Model file for the job. Use its own axes, mm. Face numbers are marked on the shaded views. A direction names the side the tool comes from. Give positions to 0.01 mm unless a question says otherwise; leave off trailing zeros. Loops run counter-clockwise (first coordinate to the right, second up) from the corner with the lowest first, then second, coordinate; pieces in that order, holes last. Notation, with made-up numbers: (28, 73) - (82, 73) arc R20 cw to (82, 92) - close; hole circle Ø8 at (37.5, -25.75). An arc over 180 degrees is marked (long way). Answer as CSV lines item,"result". Start each with the question number.
Item 1: Saw through at B-B on x = -39. Give the cut face in (y, z).
Item 2: Pin check, flat tips, straight feed: pin 1 (8 mm diameter, centred on x = -13, z = -10.5, fed in from -Y); pin 2 (4 mm diameter, centred on x = -20.5, y = 15, fed in from +Z); pin 3 (4 mm diameter, centred on x = -27, z = 18.5, fed in from -Y); pin 4 (1.5 mm diameter, centred on y = 22.5, z = -10, fed in from -X). Stop position of each tip, or through.
Item 3: Saw through at C-C on z = 0. Give the cut face in (x, y).
Item 4: Tool access for the marked faces 4, 5 and 6: list every direction of +Z, -Z, +X, -X, +Y, -Y with a clear straight run to the whole face (end or side of a thin tool).
Item 5: Saw through at A-A on z = 11. Give the cut face in (x, y).
Item 6: Drill centre lines: L1, parallel to Z at x = -61, y = 6.25; L2, parallel to Y at x = -70, z = 10; L3, parallel to X at y = 9.75, z = 12.35. Where is each one in solid material? Low to high. Write a range as from..to.
Item 7: Saw through at D-D on y = 21. Give the cut face in (x, z), plus the area to 3 significant figures.
Item 8: Pull direction X, two halves, no side cores. Call the marked faces 1, 2 and 3: pulls with the +X half, pulls with the -X half, needs draft (parallel to the pull), parting line crosses it, or undercut.
from build123d import *

# Parameters (mm, degrees)
SKETCH1_W           = 30
SKETCH1_H           = 19.5
BOSS_EXTRUDE1_DEPTH = 70
BOSS_EXTRUDE2_DEPTH = 30
SKETCH7_W           = 48
SKETCH7_H           = 45
BOSS_EXTRUDE3_DEPTH = 5
CUT_EXTRUDE2_START  = -6
SKETCH8_R           = 9.75
CUT_EXTRUDE2_DEPTH  = 18
SKETCH9_R           = 4
CUT_EXTRUDE3_DEPTH  = 92.468915485
SKETCH10_R          = 9
CUT_EXTRUDE4_DEPTH  = 10
CUT_EXTRUDE6_START  = -6
CUT_EXTRUDE6_DEPTH  = 18
FILLET1_R           = 10


with BuildPart() as part:
    # Sketch1 → Boss-Extrude1 (new body)
    with BuildSketch(Plane(origin=(0, 0, 0), x_dir=(0, 0, -1), z_dir=(1, 0, 0))):
        with Locations((0, 9.75)):
            Rectangle(SKETCH1_W, SKETCH1_H)
    extrude(amount=-BOSS_EXTRUDE1_DEPTH)

    # Sketch6 → Boss-Extrude2 (add)
    with BuildSketch(Plane.XY.offset(15)):
        with BuildLine():
            Line((-70, 19.5), (-70, 0))
            ThreePointArc((-70, 0), (-79.75, 9.75), (-70, 19.5))
        make_face()
    extrude(amount=-BOSS_EXTRUDE2_DEPTH)

    # Sketch7 → Boss-Extrude3 (add)
    with BuildSketch(Plane(origin=(0, 19.5, 0), x_dir=(1, 0, 0), z_dir=(0, 1, 0))):
        with Locations((-24, 0)):
            Rectangle(SKETCH7_W, SKETCH7_H)
    extrude(amount=BOSS_EXTRUDE3_DEPTH)

    # Sketch8 → Cut-Extrude2 (cut)
    with BuildSketch(Plane.XY.offset(15).offset(CUT_EXTRUDE2_START)):
        with Locations((-70, 9.75)):
            Circle(SKETCH8_R)
    extrude(amount=-CUT_EXTRUDE2_DEPTH, mode=Mode.SUBTRACT)

    # Sketch9 → Cut-Extrude3 (cut, through all)
    with BuildSketch(Plane.XY.offset(15)):
        with Locations((-70, 9.75)):
            Circle(SKETCH9_R)
    extrude(amount=-CUT_EXTRUDE3_DEPTH, mode=Mode.SUBTRACT)

    # Sketch10 → Cut-Extrude4 (cut)
    with BuildSketch(Plane.XZ):
        with Locations(Location((-24, 0, 0), (0, 0, 270))):
            Circle(SKETCH10_R)
    extrude(amount=-CUT_EXTRUDE4_DEPTH, mode=Mode.SUBTRACT)

    # Sketch11 → Cut-Extrude6 (cut)
    with BuildSketch(Plane(origin=(0, 0, -15), x_dir=(-1, 0, 0), z_dir=(0, 0, -1)).offset(CUT_EXTRUDE6_START)):
        Polygon((66.561504355, 11.793709299), (45, 0), (70, 0), align=None)
    extrude(amount=-CUT_EXTRUDE6_DEPTH, mode=Mode.SUBTRACT)

    # Fillet1
    fillet1_edges = [part.edges().sort_by_distance(p)[0] for p in [
        (-60.344849532, 8.393324122, 0),
    ]]
    fillet(fillet1_edges, radius=FILLET1_R)


solid = part.part
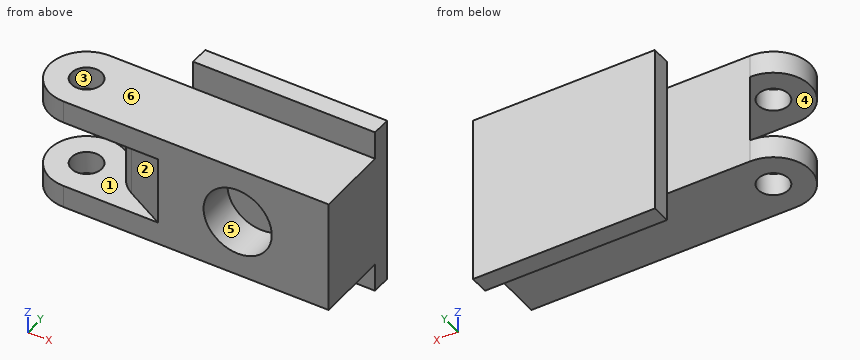
Responses:
1,outline,"(0, -15) - (19.5, -15) - (19.5, -22.5) - (24.5, -22.5) - (24.5, 22.5) - (19.5, 22.5) - (19.5, 15) - (0, 15) - close"
2,pin 1,"y = 0"
2,pin 2,"z = 15"
2,pin 3,"y = 19.5"
2,pin 4,"x = -48"
3,outline,"(-70, 19.5) arc R9.75 cw to (-60.55, 12.14) arc R10 ccw to (-55.65, 5.83) - (-45, 0) - (-33, 0) - (-33, 10) - (-15, 10) - (-15, 0) - (0, 0) - (0, 24.5) - (-48, 24.5) - (-48, 19.5) - close"
4,face 4,"-X, -Y"
4,face 5,"-Y"
4,face 6,"+Z, +X, -X, -Y"
5,outline,"(-70, 0) - (0, 0) - (0, 24.5) - (-48, 24.5) - (-48, 19.5) - (-70, 19.5) arc R9.75 ccw to start; hole circle Ø8 at (-70, 9.75)"
6,L1,"-15..-9, 9..15"
6,L2,"0..5.75, 13.75..19.5"
6,L3,"-79.75..-74, -66..0"
7,outline,"(-48, -22.5) - (0, -22.5) - (0, 22.5) - (-48, 22.5) - close"
7,area,"2,160 mm2"
8,face 1,"needs draft"
8,face 2,"pulls with the -X half"
8,face 3,"undercut"
